Build history of the part. All positions in model axes, mm. Face numbers are marked on the shaded views. A direction names the side the tool comes from. Round coordinates to 2 decimals unless told otherwise and drop trailing zeros. Order: outer loops, then holes, each group sorted by start corner. A loop starts at its lowest first (then second) coordinate and runs counter-clockwise, first axis right, second up. Notation, with made-up numbers: (56, -30.5) - (83, -30.5) arc R29 ccw to (83, -3.5) - close; hole circle Ø11 at (68.25, 31.5). An arc over 180 degrees is marked (long way). One line per question, with ' | ' between items. Start each with the question number.
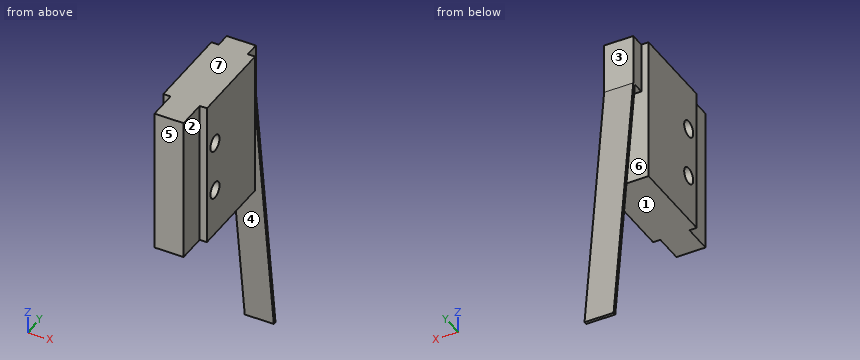
from build123d import *

# Parameters (mm, degrees)
SKETCH1_W           = 6
SKETCH1_H           = 20
BOSS_EXTRUDE1_DEPTH = 10
SKETCH3_W           = 6
SKETCH3_H           = 20
BOSS_EXTRUDE2_DEPTH = 2
SKETCH2_R           = 1.125
CUT_EXTRUDE1_DEPTH  = 7
SKETCH4_W           = 4
SKETCH4_H           = 20
BOSS_EXTRUDE3_DEPTH = 4
SKETCH5_W           = 4
SKETCH5_H           = 7
BOSS_EXTRUDE4_DEPTH = 2
BOSS_EXTRUDE5_DEPTH = 4


with BuildPart() as part:
    # Sketch1 → Boss-Extrude1 (new body)
    with BuildSketch(Plane(origin=(0, 0, 0), x_dir=(1, 0, 0), z_dir=(0, 1, 0))):
        with Locations((3, 10)):
            Rectangle(SKETCH1_W, SKETCH1_H)
    extrude(amount=BOSS_EXTRUDE1_DEPTH)

    # Sketch3 → Boss-Extrude2 (add)
    with BuildSketch(Plane(origin=(0, 0, 0), x_dir=(-1, 0, 0), z_dir=(0, -1, 0))):
        with Locations((-3, 10)):
            Rectangle(SKETCH3_W, SKETCH3_H)
    extrude(amount=BOSS_EXTRUDE2_DEPTH)

    # Sketch2 → Cut-Extrude1 (cut)
    with BuildSketch(Plane(origin=(6, 0, 0), x_dir=(0, 0, -1), z_dir=(1, 0, 0))):
        with Locations((6.5, 0)):
            Circle(SKETCH2_R)
        with Locations((13.5, 0)):
            Circle(SKETCH2_R)
    extrude(amount=-CUT_EXTRUDE1_DEPTH, mode=Mode.SUBTRACT)

    # Sketch4 → Boss-Extrude3 (add)
    with BuildSketch(Plane(origin=(0, -2, 0), x_dir=(-1, 0, 0), z_dir=(0, -1, 0))):
        with Locations((-3, 10)):
            Rectangle(SKETCH4_W, SKETCH4_H)
    extrude(amount=BOSS_EXTRUDE3_DEPTH)

    # Sketch5 → Boss-Extrude4 (add)
    with BuildSketch(Plane(origin=(0, 10, 0), x_dir=(1, 0, 0), z_dir=(0, 1, 0))):
        with Locations((3, 3.5)):
            Rectangle(SKETCH5_W, SKETCH5_H)
    extrude(amount=BOSS_EXTRUDE4_DEPTH)

    # Sketch7 → Boss-Extrude5 (add)
    with BuildSketch(Plane(origin=(5, 0, 0), x_dir=(0, 0, -1), z_dir=(1, 0, 0))):
        Polygon((7, 12), (44.5, 16.9), (44.5, 16.491160733), (7, 11.591160733), (7, 10), (0, 10), (0, 12), align=None)
    extrude(amount=-BOSS_EXTRUDE5_DEPTH)


solid = part.part
Item 1: 3-axis set-ups, long thin cutter, end or side, ignore diameter. For the marked faces 1, 2 and 3: which of +Z, -Z, +X, -X, +Y, -Y reach the whole face in a straight line?
Item 2: Slice it at D-D (z = -13.5). Write the cut outline in (x, y) (1 decimal), plus the area to 3 significant figures.
Item 3: Slice it at C-C (x = 1.75). Write the cut outline in (y, z) (3 decimals).
Item 4: Pull direction Y, two halves, no side cores. Call the marked faces 4, 5, 6 and 7: released by +Y, released by -Y, zero draft, split by the parting line, or undercut.
Item 5: Pin check, flat tips, straight feed: pin 1 (1.3 mm diameter, centred on x = 2, y = 10.5, fed in from -Z); pin 2 (1.8 mm diameter, centred on x = 4, z = -10, fed in from +Y); pin 3 (2 mm diameter, centred on x = 3, z = -2, fed in from +Y). Stop position of each tip, or through.
Item 6: Wall check: line 1 along Y through (x, z) = (4.1, -6.5) (3 decimals); line 2 along Z through (x, y) = (2.85, 10.25); line 3 along X through (y, z) = (12.5, -12). Give the ranges that are in metal, low to high. Write a range as [from, to].
Item 7: Slice it at A-A (y = 0). Write the cut outline in (x, z) (3 decimals).
Item 8: Slice it at B-B (z = -6.5). Write the cut outline in (x, y) (3 decimals).
A:
1) face 1: -Z, +X, -X, -Y | face 2: +Z, -Z, +X, -Y | face 3: +Z, +X, -X, +Y
2) outline: (0, -2) - (1, -2) - (1, -6) - (5, -6) - (5, -2) - (6, -2) - (6, -1.1) - (0, -1.1) - close; (0, 1.1) - (6, 1.1) - (6, 10) - (0, 10) - close; (1, 12.4) - (5, 12.4) - (5, 12.8) - (1, 12.8) - close | area: 76.1 mm^2
3) outline: (-6, -20) - (10, -20) - (10, -7) - (11.591, -7) - (16.491, -44.5) - (16.9, -44.5) - (12, -7) - (12, 0) - (-6, 0) - close; hole circle Ø2.25 at (0, -13.5); hole circle Ø2.25 at (0, -6.5)
4) face 4: undercut | face 5: released by -Y | face 6: undercut | face 7: zero draft
5) pin 1: z = -20 | pin 2: y = 12.51 | pin 3: y = 12
6) line 1: [-6, -1.125], [1.125, 12] | line 2: [-7, 0] | line 3: [1, 5]
7) outline: (0, -20) - (6, -20) - (6, -14.625) - (0, -14.625) - close; (0, -12.375) - (6, -12.375) - (6, -7.625) - (0, -7.625) - close; (0, -5.375) - (6, -5.375) - (6, 0) - (0, 0) - close
8) outline: (0, -2) - (1, -2) - (1, -6) - (5, -6) - (5, -2) - (6, -2) - (6, -1.125) - (0, -1.125) - close; (0, 1.125) - (6, 1.125) - (6, 10) - (5, 10) - (5, 12) - (1, 12) - (1, 10) - (0, 10) - close
